Can you work these out from the model? Positions are in its coordinate system, mm. Coordinates: 2 decimals unless noted, no trailing zeros. Order: outer loops, then holes, each group sorted by start corner. A loop starts at its lowest first (then second) coordinate and runs counter-clockwise, first axis right, second up. Notation, with made-up numbers: M 67,-25.75 L 104,-25.75 A29 ccw 104,-2.75 Z; hole C 11.25,19.25 d6. An arc over 180 degrees is marked long. Answer as CSV lines item,"result". Start each with the question number.
1. If we section it at C-C (z = -92): List the corners of the cut face in (x, y) for me.
2. If we section it at A-A (y = 1): Give the number of separate pieces and of enclosed holes in the cut face, plus the area to 3 significant figures.
3. I need wall thicknesses on line 1 along Z through (x, y) = (0, 2.15); line 2 along X through (y, z) = (2, 152); line 3 along X through (y, z) = (1, 57). Which ranges of each line are inside material? Lowest first, please. Write a range as from..to.
4. If we section it at B-B (x = 205): List the corners of the cut face in (y, z) for me.
5. Will these pins go through, and if not, where does the flat tip stop? pin 1 (1 mm diameter, centred on y = 1, z = 188, fed in from +X); pin 2 (2.5 mm diameter, centred on x = -111.68, z = -153.71, fed in from -Y); pin 3 (1 mm diameter, centred on x = -67, y = 1, fed in from +Z); pin 4 (1.5 mm diameter, centred on x = -90, y = 0.5, fed in from -Z).
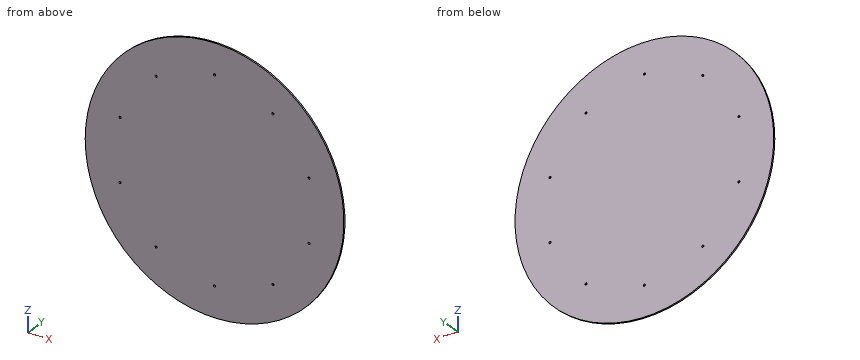
Autodesk Inventor part; units mm, degrees
ref_plane "YZ Plane" through (0, 0, 0) normal (1, 0, 0) x (0, 1, 0)
ref_plane "XZ Plane" through (0, 0, 0) normal (0, 1, 0) x (-1, 0, 0)
ref_plane "XY Plane" through (0, 0, 0) normal (0, 0, 1) x (1, 0, 0)
sketch "Skizze1" plane through (0, 0, 0) normal (0, 1, 0) x (-1, 0, 0)
  circle A0 centre (0, 0) radius 247.5
  dimension "d0" = 495
extrude "Extrusion_grundplatte" add sketch "Skizze1" along normal blind 3
sketch "Skizze6" plane through (0, 0, 0) normal (0, -1, 0) x (1, 0, 0)
  circle A0 centre (0, 0) radius 247.5
  line L0 (0, 0) -> (0, 190) construction
  line L1 (0, 0) -> (-111.6792, 153.7132) construction
  line L2 (0, 0) -> (-180.7007, 58.7132) construction
  line L3 (0, 0) -> (-180.7007, -58.7132) construction
  line L4 (0, 0) -> (-111.6792, -153.7132) construction
  line L5 (0, 0) -> (0, -190) construction
  line L6 (0, 0) -> (111.6792, -153.7132) construction
  line L7 (0, 0) -> (180.7007, -58.7132) construction
  line L8 (0, 0) -> (180.7007, 58.7132) construction
  line L9 (0, 0) -> (111.6792, 153.7132) construction
  dimension "d47" = 190
  dimension "d50" = 360
hole "Bohrung_halter_plexiglas" at (0, 0, 190) at (-111.6792, 0, 153.7132) at (-180.7007, 0, 58.7132) at (-180.7007, 0, -58.7132) at (-111.6792, 0, -153.7132) at (0, 0, -190) at (111.6792, 0, -153.7132) at (180.7007, 0, -58.7132) at (180.7007, 0, 58.7132) at (111.6792, 0, 153.7132) direction (0, 1, 0) diameter 4 end through all
properties part number "Plexiglas" material "Plexiglas"
Solved:
1,outline,"M -229.77,0 L 229.77,0 L 229.77,3 L -229.77,3 Z"
2,separate pieces,"1"
2,enclosed holes,"10"
2,area,"192,000 mm²"
3,line 1,"-247.5..-192, -188..188, 192..247.5"
3,line 2,"-195.33..-112.71, -110.65..110.65, 112.71..195.33"
3,line 3,"-240.85..-181.73, -179.67..179.67, 181.73..240.85"
4,outline,"M 0,-138.68 L 3,-138.68 L 3,138.68 L 0,138.68 Z"
5,pin 1,"x = 161.55"
5,pin 2,"through"
5,pin 3,"z = 238.4"
5,pin 4,"z = -230.85"
